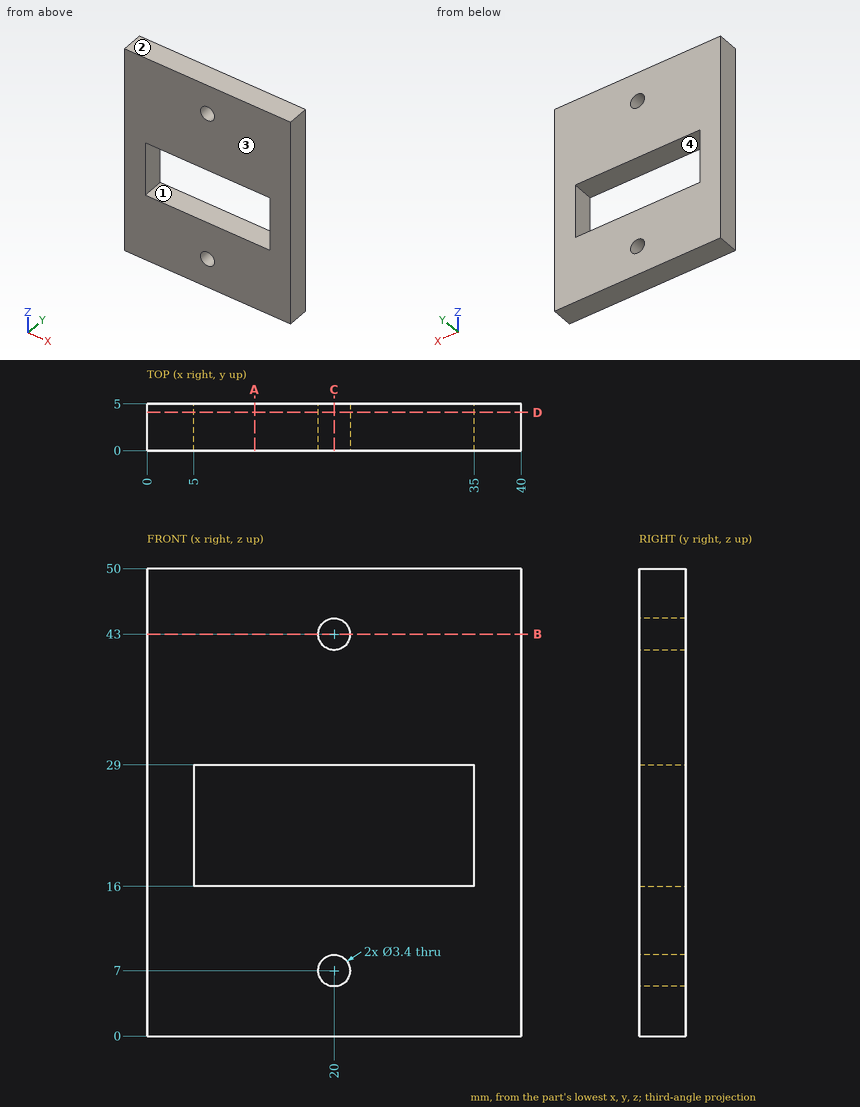
Design review of the part shown in the three views and the two pictorial views. Dimensions are in mm from the part's minimum x, y and z. A direction names the side the tool comes from. Give positions to 0.01 mm unless a question says otherwise; leave off trailing zeros. Loops run counter-clockwise (first coordinate to the right, second up) from the corner with the lowest first, then second, coordinate; pieces in that order, holes last. Notation, with made-up numbers: (25.5, 88) - (76.5, 88) arc R25 ccw to (76.5, 112) - close; hole circle Ø9 at (-23, 27). An arc over 180 degrees is marked (long way). Answer as a JSON object with one key per item and string values.
Q1. For the marked faces 1 and 2, list the 3-axis set-ups (+Z, -Z, +X, -X, +Y, -Y) from which the entire face can be reached by the end or side of a thin tool; tool diameter is ignored.
Worked out:
{"face 1": "+Y, -Y", "face 2": "+Z, +X, -X, +Y, -Y"}
Q2. Add section C-C on x = 20. State the section outline as (y, z) points.
Worked out:
{"outline": "(0, 0) - (5, 0) - (5, 5.3) - (0, 5.3) - close; (0, 8.7) - (5, 8.7) - (5, 16) - (0, 16) - close; (0, 29) - (5, 29) - (5, 41.3) - (0, 41.3) - close; (0, 44.7) - (5, 44.7) - (5, 50) - (0, 50) - close"}
Q3. Add section D-D on y = 4.1. State the section outline as (x, z) points, plus the area to 3 significant figures.
Worked out:
{"outline": "(0, 0) - (40, 0) - (40, 50) - (0, 50) - close; hole (5, 16) - (35, 16) - (35, 29) - (5, 29) - close; hole circle Ø3.4 at (20, 7); hole circle Ø3.4 at (20, 43)", "area": "1,590 mm^2"}
Q4. Add section A-A on x = 11.5. State the section outline as (y, z) points.
Worked out:
{"outline": "(0, 0) - (5, 0) - (5, 16) - (0, 16) - close; (0, 29) - (5, 29) - (5, 50) - (0, 50) - close"}
Q5. Add section B-B on z = 43. State the section outline as (x, y) points.
Worked out:
{"outline": "(0, 0) - (18.3, 0) - (18.3, 5) - (0, 5) - close; (21.7, 0) - (40, 0) - (40, 5) - (21.7, 5) - close"}
Q6. To check wall thickness, follow line 1 along Z through (x, y) = (20, 2.65); line 2 along Z through (x, y) = (29.5, 4.75); line 3 along Z through (x, y) = (19.5, 0.2). State the ranges of each line that lie inside material, in increasing order.
Worked out:
{"line 1": "z = 0 to 5.3, 8.7 to 16, 29 to 41.3, 44.7 to 50", "line 2": "z = 0 to 16, 29 to 50", "line 3": "z = 0 to 5.38, 8.62 to 16, 29 to 41.38, 44.62 to 50"}
Q7. Mouldability with a two-part tool opening along X and no side actions: class the marked faces 3 and 4 as +X half, -X half, draft (parallel to the pull), parting line (faces both ways), or undercut.
Worked out:
{"face 3": "draft", "face 4": "undercut"}
